from build123d import *

# Parameters (mm, degrees)
SKETCH1_W            = 49.5
SKETCH1_H            = 22
BOSS_EXTRUDE1_DEPTH  = 3.175
SKETCH2_W            = 30
SKETCH2_H            = 22
BOSS_EXTRUDE2_DEPTH  = 2.8
FILLET1_R            = 5
SKETCH4_W            = 27
SKETCH4_H            = 19.2
BOSS_EXTRUDE3_DEPTH  = 12.5
CHAMFER1_SIZE        = 5
FILLET2_R            = 4
SKETCH3_R            = 1.7
CUT_EXTRUDE1_DEPTH   = 16.675
CUT_EXTRUDE2_DEPTH   = 16.2
MIRROR2_COPY_1_DEPTH = 16.2
CHAMFER2_SIZE        = 1.3
CUT_EXTRUDE4_DEPTH   = 17
FILLET3_R            = 4
SKETCH9_W            = 5.3
SKETCH9_H            = 11.15
BOSS_EXTRUDE4_DEPTH  = 1
SKETCH10_W           = 0.75
SKETCH10_H           = 6.5
BOSS_EXTRUDE5_DEPTH  = 9.22
CHAMFER3_SIZE        = 1
CUT_EXTRUDE3_DEPTH   = 2


with BuildPart() as part:
    # Sketch1 → Boss-Extrude1 (new body)
    with BuildSketch(Plane.XY):
        Rectangle(SKETCH1_W, SKETCH1_H)
    extrude(amount=BOSS_EXTRUDE1_DEPTH)

    # Sketch2 → Boss-Extrude2 (add)
    with BuildSketch(Plane.XY.offset(3.175)):
        Rectangle(SKETCH2_W, SKETCH2_H)
    extrude(amount=BOSS_EXTRUDE2_DEPTH)

    # Fillet1
    fillet1_edges = [part.edges().sort_by_distance(p)[0] for p in [
        (-15, 11, 4.575),
        (15, 11, 4.575),
        (15, -11, 4.575),
        (-15, -11, 4.575),
    ]]
    fillet(fillet1_edges, radius=FILLET1_R)

    # Sketch4 → Boss-Extrude3 (add)
    with BuildSketch(Plane(origin=(0, 0, 0), x_dir=(-1, 0, 0), z_dir=(0, 0, -1))):
        Rectangle(SKETCH4_W, SKETCH4_H)
    extrude(amount=BOSS_EXTRUDE3_DEPTH)

    # Chamfer1
    chamfer1_edges = [part.edges().sort_by_distance(p)[0] for p in [
        (13.5, 9.6, -6.25),
        (-13.5, 9.6, -6.25),
    ]]
    chamfer(chamfer1_edges, length=CHAMFER1_SIZE)

    # Fillet2
    fillet2_edges = [part.edges().sort_by_distance(p)[0] for p in [
        (13.5, -9.6, -6.25),
        (-13.5, -9.6, -6.25),
        (8.5, 9.6, -6.25),
        (-8.5, 9.6, -6.25),
        (-13.5, 4.6, -6.25),
        (13.5, 4.6, -6.25),
    ]]
    fillet(fillet2_edges, radius=FILLET2_R)

    # Sketch3 → Cut-Extrude1 (cut, through all)
    with BuildSketch(Plane.XY.offset(3.175)):
        with Locations((-20, 0)):
            Circle(SKETCH3_R)
        with Locations((20, 0)):
            Circle(SKETCH3_R)
    extrude(amount=-CUT_EXTRUDE1_DEPTH, mode=Mode.SUBTRACT)

    # Sketch5 → Cut-Extrude2 (cut)
    with BuildSketch(Plane.XY.offset(3.175)):
        with BuildLine():
            Line((-12.426380479, 10.371804865), (-21.661656574, 5.246165837))
            ThreePointArc((-21.661656574, 5.246165837), (-23.92058698, 3.043851225), (-24.75, 0))
            Line((-24.75, 0), (-24.75, 11))
            Line((-24.75, 11), (-10, 11))
            ThreePointArc((-10, 11), (-11.253191062, 10.840404132), (-12.426380479, 10.371804865))
        make_face()
    cut_extrude2 = extrude(amount=-CUT_EXTRUDE2_DEPTH, mode=Mode.SUBTRACT)

    # Mirror1: Cut-Extrude2 across plane
    add(cut_extrude2.mirror(Plane.ZX), mode=Mode.SUBTRACT)

    # Mirror2: Cut-Extrude2 across plane
    add(cut_extrude2.mirror(Plane(origin=(0, 0, 0), x_dir=(0, 0, 1), z_dir=(1, 0, 0))), mode=Mode.SUBTRACT)

    # Mirror2 copy 1 sketch → Mirror2 copy 1 (cut)
    with BuildSketch(Plane(origin=(0, 0, 3.175), x_dir=(-1, 0, 0), z_dir=(0, 0, 1))):
        with BuildLine():
            Line((-12.426380479, 10.371804865), (-21.661656574, 5.246165837))
            ThreePointArc((-21.661656574, 5.246165837), (-23.92058698, 3.043851225), (-24.75, 0))
            Line((-24.75, 0), (-24.75, 11))
            Line((-24.75, 11), (-10, 11))
            ThreePointArc((-10, 11), (-11.253191062, 10.840404132), (-12.426380479, 10.371804865))
        make_face()
    extrude(amount=-MIRROR2_COPY_1_DEPTH, mode=Mode.SUBTRACT)

    # Chamfer2
    chamfer2_edges = [part.edges().sort_by_distance(p)[0] for p in [
        (-21.7, 0, 3.175),
        (18.3, 0, 3.175),
    ]]
    chamfer(chamfer2_edges, length=CHAMFER2_SIZE)

    # Sketch8 → Cut-Extrude4 (cut)
    with BuildSketch(Plane.XY.offset(5.975)):
        with BuildLine():
            Line((-7.25, 8.25), (-12.25, 3.25))
            Line((-12.25, 3.25), (-12.25, -6))
            ThreePointArc((-12.25, -6), (-11.590990258, -7.590990258), (-10, -8.25))
            Line((-10, -8.25), (10, -8.25))
            ThreePointArc((10, -8.25), (11.590990258, -7.590990258), (12.25, -6))
            Line((12.25, -6), (12.25, 3.25))
            Line((12.25, 3.25), (7.25, 8.25))
            Line((7.25, 8.25), (-7.25, 8.25))
        make_face()
    extrude(amount=-CUT_EXTRUDE4_DEPTH, mode=Mode.SUBTRACT)

    # Fillet3
    fillet3_edges = [part.edges().sort_by_distance(p)[0] for p in [
        (-7.25, 8.25, -2.525),
        (7.25, 8.25, -2.525),
        (12.25, 3.25, -2.525),
        (-12.25, 3.25, -2.525),
    ]]
    fillet(fillet3_edges, radius=FILLET3_R)

    # Sketch9 → Boss-Extrude4 (add)
    with BuildSketch(Plane(origin=(0, 0, -12.5), x_dir=(-1, 0, 0), z_dir=(0, 0, -1))):
        with Locations((0, 3.525)):
            Rectangle(SKETCH9_W, SKETCH9_H)
        with Locations((-7.05, -3.525)):
            Rectangle(SKETCH9_W, SKETCH9_H)
        with Locations((7.05, -3.525)):
            Rectangle(SKETCH9_W, SKETCH9_H)
    extrude(amount=BOSS_EXTRUDE4_DEPTH)

    # Sketch10 → Boss-Extrude5 (add)
    with BuildSketch(Plane(origin=(0, 0, -13.5), x_dir=(-1, 0, 0), z_dir=(0, 0, -1))):
        with Locations((0, 3.525)):
            Rectangle(SKETCH10_W, SKETCH10_H)
        with Locations((-7.05, -3.525)):
            Rectangle(SKETCH10_W, SKETCH10_H)
        with Locations((7.05, -3.525)):
            Rectangle(SKETCH10_W, SKETCH10_H)
    extrude(amount=BOSS_EXTRUDE5_DEPTH)

    # Chamfer3
    chamfer3_edges = [part.edges().sort_by_distance(p)[0] for p in [
        (0, 0.275, -22.72),
        (0, 6.775, -22.72),
        (7.05, -6.775, -22.72),
        (7.05, -0.275, -22.72),
        (-7.05, -6.775, -22.72),
        (-7.05, -0.275, -22.72),
    ]]
    chamfer(chamfer3_edges, length=CHAMFER3_SIZE)

    # Sketch6 → Cut-Extrude3 (cut)
    with BuildSketch(Plane.XY.offset(5.975)):
        with BuildLine():
            Line((-13.5, 6), (-13.5, -6))
            ThreePointArc((-13.5, -6), (-12.474873734, -8.474873734), (-10, -9.5))
            Line((-10, -9.5), (10, -9.5))
            ThreePointArc((10, -9.5), (12.474873734, -8.474873734), (13.5, -6))
            Line((13.5, -6), (13.5, 6))
            ThreePointArc((13.5, 6), (12.474873734, 8.474873734), (10, 9.5))
            Line((10, 9.5), (-10, 9.5))
            ThreePointArc((-10, 9.5), (-12.474873734, 8.474873734), (-13.5, 6))
        make_face()
    extrude(amount=-CUT_EXTRUDE3_DEPTH, mode=Mode.SUBTRACT)


solid = part.part
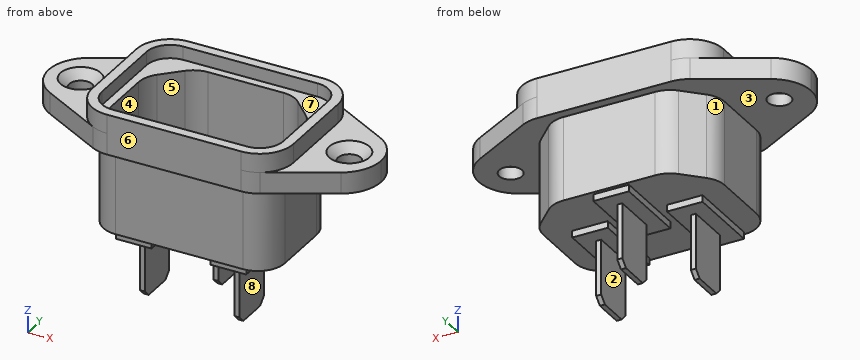
Geometry: final body of the model. Coordinates: model frame, mm. Face numbers are marked on the shaded views. A direction names the side the tool comes from. Give positions to 0.01 mm unless a question says otherwise; leave off trailing zeros. Write each loop counter-clockwise with the first axis right and the second up, starting at its lowest first coordinate (ties: lowest second). Pieces come first, ordered by that corner, then holes. Notation, with made-up numbers: M 27.5,-6 L 64.5,-6 A22 cw 64.5,3 Z; hole C 84.5,-21 d4. An arc over 180 degrees is marked long. Answer in a Markdown table with one row per item. Add a question column.
(1) Section A-A on z = -2.5. Return loops of the section in (x, y), and give its area (3 significant figures).
(2) First-contact query: pin 1 (8 mm diameter, centred on x = -6, y = 4.5, fed in from +Z) (3 decimals); pin 2 (2 mm diameter, centred on y = 2, z = -17, fed in from +X) (3 decimals); pin 3 (0.8 mm diameter, centred on x = -7, z = -19, fed in from -Y) (3 decimals); pin 4 (8.5 mm diameter, centred on y = -3, z = -1, fed in from -X). Flat tips, straight axial feed; report the tip coordinate or a pass-through.
(3) Ray query, line 1 (Y direction, x = 5.5, z = -7.5); line 2 (X direction, y = -3.5, z = -4); line 3 (X direction, y = -5.25, z = -21.5) (3 decimals). Return the intervals inside material, ascending.
(4) Section D-D on x = 3.5. Return loops of the section in (y, z) (3 decimals), and give its area (4 significant figures).
(5) Section B-B on x = -2. Return loops of the section in (y, z) (3 decimals).
(6) Reachability of the marked faces 1, 2, 3 and 4 from +Z, -Z, +X, -X, +Y, -Y: full face, straight path, thin tool, end or side. Return the list, or none.
(7) Section C-C on x = 20. Return loops of the section in (y, z) (3 decimals), and give its area (3 significant figures).
(8) Mould query, pull axis Y, two halves, no side actions, for the marked faces 5, 6, 7 and 8. Classes: +Y half, -Y half, draft (parallel to the pull), parting line (faces both ways), or undercut.
Result set:
| question | item | result |
|---|---|---|
| 1 | outline | M -13.5,-5.6 A4 ccw -9.5,-9.6 L 9.5,-9.6 A4 ccw 13.5,-5.6 L 13.5,2.94 A4 ccw 12.33,5.77 L 9.67,8.43 A4 ccw 6.84,9.6 L -6.84,9.6 A4 ccw -9.67,8.43 L -12.33,5.77 A4 ccw -13.5,2.94 Z; hole M -12.25,-6 A2.25 ccw -10,-8.25 L 10,-8.25 A2.25 ccw 12.25,-6 L 12.25,1.59 A4 ccw 11.08,4.42 L 8.42,7.08 A4 ccw 5.59,8.25 L -5.59,8.25 A4 ccw -8.42,7.08 L -11.08,4.42 A4 ccw -12.25,1.59 Z |
| 1 | area | 109 mm^2 |
| 2 | pin 1 | stops at z = 3.975 |
| 2 | pin 2 | stops at x = 0.375 |
| 2 | pin 3 | stops at y = -6.775 |
| 2 | pin 4 | stops at x = -24.75 |
| 3 | line 1 | y = -9.6 to -8.25, 8.25 to 9.6 |
| 3 | line 2 | x = -13.5 to -12.25, 12.25 to 13.5 |
| 3 | line 3 | x = -7.425 to -6.675, 6.675 to 7.425 |
| 4 | outline | M -11,0 L -9.6,0 L -9.6,-12.5 L 9.6,-12.5 L 9.6,0 L 11,0 L 11,5.975 L 9.5,5.975 L 9.5,3.975 L 8.25,3.975 L 8.25,-11.025 L -8.25,-11.025 L -8.25,3.975 L -9.5,3.975 L -9.5,5.975 L -11,5.975 Z |
| 4 | area | 85.95 mm^2 |
| 5 | outline | M -11,0 L -9.6,0 L -9.6,-12.5 L -2.05,-12.5 L -2.05,-13.5 L 9.1,-13.5 L 9.1,-12.5 L 9.6,-12.5 L 9.6,0 L 11,0 L 11,5.975 L 9.5,5.975 L 9.5,3.975 L 8.25,3.975 L 8.25,-11.025 L -8.25,-11.025 L -8.25,3.975 L -9.5,3.975 L -9.5,5.975 L -11,5.975 Z |
| 6 | face 1 | -Z, -X, +Y |
| 6 | face 2 | -Z, +Y, -Y |
| 6 | face 3 | -Z |
| 6 | face 4 | +Z |
| 7 | outline | M -6.168,0 L -1.7,0 L -1.7,1.875 L -3,3.175 L -6.168,3.175 Z; M 1.7,0 L 6.168,0 L 6.168,3.175 L 3,3.175 L 1.7,1.875 Z |
| 7 | area | 26.7 mm^2 |
| 8 | face 5 | undercut |
| 8 | face 6 | -Y half |
| 8 | face 7 | undercut |
| 8 | face 8 | draft |
